The figure shows three views and two pictorial views of one solid part (mm, origin at its lowest corner). Answer the questions. A direction names the side the tool comes from. Coordinates: 2 decimals unless noted, no trailing zeros. Write each loop counter-clockwise with the first axis right and the second up, starting at its lowest first coordinate (ties: lowest second). Pieces come first, ordered by that corner, then holes.
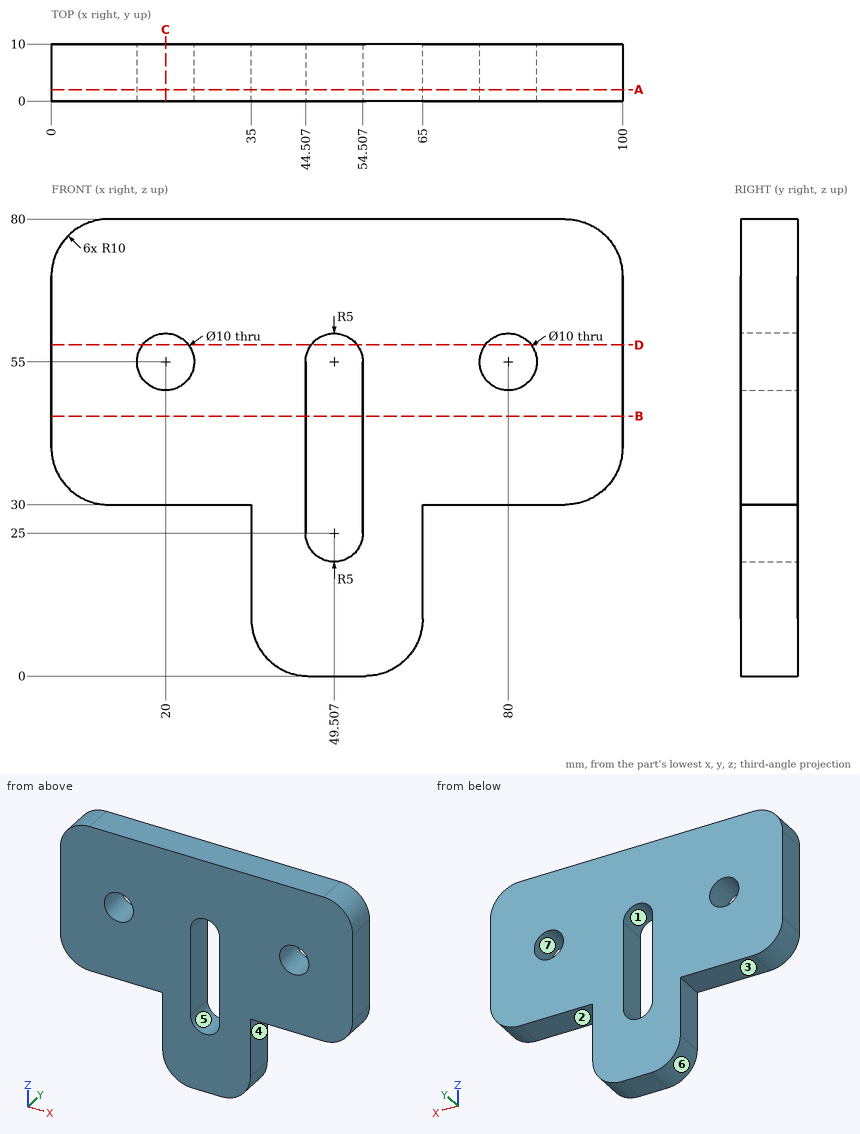
1. Section D-D on z = 58 is taken. Give the vertices of the cut face in (x, y), then the cut area to 3 significant figures.
Results found:
outline: (0, 0) - (16, 0) - (16, 10) - (0, 10) - close; (24, 0) - (45.51, 0) - (45.51, 10) - (24, 10) - close; (53.51, 0) - (76, 0) - (76, 10) - (53.51, 10) - close; (84, 0) - (100, 0) - (100, 10) - (84, 10) - close
area: 760 mm2
2. Section B-B on z = 45.5 is taken. Give the vertices of the cut face in (x, y), then the cut area to 3 significant figures.
Results found:
outline: (0, 0) - (44.51, 0) - (44.51, 10) - (0, 10) - close; (54.51, 0) - (100, 0) - (100, 10) - (54.51, 10) - close
area: 900 mm2
3. Flat-ended cylindrical pins translate along their axes: P1, Ø6, axis at x = 20, z = 55, coming from the +Y side; P2, Ø3, axis at x = 57, y = 2, coming from the -Z side; P3, Ø11.5, axis at x = 80, z = 55, coming from the +Y side; P4, Ø1, axis at x = 23, y = 5.5, coming from the -Z side. Find the tip coordinate at first contact, or state that the pin passes through.
Results found:
P1: passes through
P2: stops at z = 0.01
P3: stops at y = 10
P4: stops at z = 30
4. Section C-C on x = 20 is taken. Give the vertices of the cut face in (y, z).
Results found:
outline: (0, 30) - (10, 30) - (10, 50) - (0, 50) - close; (0, 60) - (10, 60) - (10, 80) - (0, 80) - close
5. Section A-A on y = 2 is taken. Give the vertices of the cut face in (x, z), then the cut area to 3 significant figures.
Results found:
outline: (0, 40) arc R10 ccw to (10, 30) - (35, 30) - (35, 10) arc R10 ccw to (45, 0) - (55, 0) arc R10 ccw to (65, 10) - (65, 30) - (90, 30) arc R10 ccw to (100, 40) - (100, 70) arc R10 ccw to (90, 80) - (10, 80) arc R10 ccw to (0, 70) - close; hole circle Ø10 at (20, 55); hole (44.51, 25) arc R5 ccw to (54.51, 25) - (54.51, 55) arc R5 ccw to (44.51, 55) - close; hole circle Ø10 at (80, 55)
area: 5,240 mm2
6. A tool of negligible diameter and unlimited length cuts with its end or side. For the marked faces 1, 2 and 3, from which of +Z, -Z, +X, -X, +Y, -Y can it reach the whole face along a straight path? Write none if from no direction.
Results found:
face 1: +Y, -Y
face 2: -Z, +X, +Y, -Y
face 3: -Z, -X, +Y, -Y
7. For a pull along Z with two mould halves and no side action, classify the marked faces 4, 5, 6 and 7 as pulls with the +Z half, pulls with the -Z half, needs draft (parallel to the pull), parting line crosses it, or undercut.
Results found:
face 4: needs draft
face 5: undercut
face 6: pulls with the -Z half
face 7: undercut
8. Find the intervals of material crossed by L1, parallel to X at y = 2, z = 55; L2, parallel to Z at x = 20, y = 3.25; L3, parallel to X at y = 9.75, z = 48, in increasing order.
Results found:
L1: x = 0 to 15, 25 to 44.51, 54.51 to 75, 85 to 100
L2: z = 30 to 50, 60 to 80
L3: x = 0 to 44.51, 54.51 to 100
